from build123d import *

# Parameters (mm, degrees)
SKETCH1_R                      = 29.464
BASE_DEPTH                     = 25.4
SKETCH2_W                      = 33.02
SKETCH2_H                      = 3.81
A_ARMS_DEPTH                   = 25.4
FILLET_A_ARM_TAB_F_R           = 16.51
FILLET2_R                      = 50.8
BOSS_EXTRUDE3_DEPTH            = 10
FILLET3_R                      = 12.7
SKETCH6_R                      = 4.064
TAB_HOLES_1_DEPTH              = 38.1
SKETCH7_R                      = 4.064
TAB_HOLES_2_DEPTH              = 177.509801452
MID_FEATURE_BEARING_DEPTH      = 1.524
MID_FEATURE_BEARING_DEPTH_BACK = 1.524
SKETCH8_R                      = 29.464
SKETCH8_R_2                    = 26.924
SKETCH11_R                     = 4.318
TAB_HOLES_3_DEPTH              = 50.8


with BuildPart() as part:
    # Sketch1 → Base (new body)
    with BuildSketch(Plane(origin=(0, 0, 0), x_dir=(1, 0, 0), z_dir=(0, 1, 0))):
        with BuildLine():
            Line((-58.88559997, -79.728413598), (36.107103946, -79.728413598))
            Line((36.107103946, -79.728413598), (42.479503863, -4.99030836))
            Line((42.479503863, -4.99030836), (36.107103946, 103.339537331))
            Line((36.107103946, 103.339537331), (9.149946216, 103.339537331))
            ThreePointArc((9.149946216, 103.339537331), (-6.239768533, 98.146384684), (-15.336480298, 84.690457011))
            Line((-15.336480298, 84.690457011), (-53.313910816, -53.058413598))
            Line((-53.313910816, -53.058413598), (-58.88559997, -53.058413598))
            Line((-58.88559997, -53.058413598), (-58.88559997, -79.728413598))
        make_face()
        with Locations(Location((0, 0, 0), (0, 0, 270))):
            Circle(SKETCH1_R, mode=Mode.SUBTRACT)
    extrude(amount=BASE_DEPTH)

    # Sketch2 → A-Arms (add)
    with BuildSketch(Plane(origin=(0, 0, 0), x_dir=(1, 0, 0), z_dir=(0, 1, 0))):
        Polygon((36.107103946, 103.339537331), (36.331223565, 99.529537331), (3.087103946, 99.529537331), (3.087103946, 103.339537331), align=None)
        Polygon((3.087103946, -75.918413598), (36.431956223, -75.918413598), (36.107103946, -79.728413598), (3.087103946, -79.728413598), align=None)
        Polygon((3.087103946, 80.479537331), (3.087103946, 76.669537331), (37.675941275, 76.669537331), (37.451821657, 80.479537331), align=None)
        Polygon((3.087103946, -53.058413598), (38.381069887, -53.058413598), (38.056217609, -56.868413598), (3.087103946, -56.868413598), align=None)
        with Locations((-42.37559997, -54.963413598)):
            Rectangle(SKETCH2_W, SKETCH2_H)
        with Locations((-42.37559997, -77.823413598)):
            Rectangle(SKETCH2_W, SKETCH2_H)
    extrude(amount=-A_ARMS_DEPTH)

    # Fillet a-arm tab f
    # the kernel refuses this fillet: 16.51 mm, written as the material it takes off along each edge
    with BuildSketch(Plane(origin=(39.93846651, -25.4, 34.792630802), x_dir=(-0.9963848042708363, 0, -0.08495482221844149), z_dir=(-0.08495482221844149, 0, 0.9963848042708364)), Plane(origin=(41.887580174, -25.4, 11.932630802), x_dir=(-0.9963848042708365, 0, -0.08495482221843932), z_dir=(-0.08495482221843934, 0, 0.9963848042708366))) as fillet_a_arm_tab_f_piece_1:
        with BuildLine():
            CenterArc((FILLET_A_ARM_TAB_F_R, -FILLET_A_ARM_TAB_F_R), FILLET_A_ARM_TAB_F_R, 90, 90)
            Line((0, -FILLET_A_ARM_TAB_F_R), (0, 0))
            Line((0, 0), (FILLET_A_ARM_TAB_F_R, 0))
        make_face()
    extrude(amount=86.373823872, mode=Mode.SUBTRACT)
    with BuildSketch(Plane(origin=(3.087103946, -25.4, 121.003413598), x_dir=(0, 1, 0), z_dir=(0, 0, -1)), Plane(origin=(3.087103946, -25.4, -121.754537331), x_dir=(1, 0, 0), z_dir=(0, 0, 1)), Plane(origin=(-25.86559997, -25.4, 98.143413598), x_dir=(-1, 0, 0), z_dir=(0, 0, -1)), Plane(origin=(-58.88559997, -25.4, 11.783413598), x_dir=(1, 0, 0), z_dir=(0, 0, 1))) as fillet_a_arm_tab_f_piece_2:
        with BuildLine():
            CenterArc((FILLET_A_ARM_TAB_F_R, FILLET_A_ARM_TAB_F_R), FILLET_A_ARM_TAB_F_R, 180, 90)
            Line((0, FILLET_A_ARM_TAB_F_R), (0, 0))
            Line((0, 0), (FILLET_A_ARM_TAB_F_R, 0))
        make_face()
    extrude(amount=86.36, mode=Mode.SUBTRACT)
    with BuildSketch(Plane(origin=(3.087103946, -25.4, 98.143413598), x_dir=(1, 0, 0), z_dir=(0, 0, -1)), Plane(origin=(3.087103946, -25.4, -58.254537331), x_dir=(1, 0, 0), z_dir=(0, 0, -1)), Plane(origin=(-58.88559997, -25.4, 121.003413598), x_dir=(1, 0, 0), z_dir=(0, 0, -1)), Plane(origin=(-25.86559997, -25.4, 34.643413598), x_dir=(-1, 0, 0), z_dir=(0, 0, 1))) as fillet_a_arm_tab_f_piece_3:
        with BuildLine():
            CenterArc((FILLET_A_ARM_TAB_F_R, -FILLET_A_ARM_TAB_F_R), FILLET_A_ARM_TAB_F_R, 90, 90)
            Line((0, -FILLET_A_ARM_TAB_F_R), (0, 0))
            Line((0, 0), (FILLET_A_ARM_TAB_F_R, 0))
        make_face()
    extrude(amount=86.36, mode=Mode.SUBTRACT)
    with BuildSketch(Plane(origin=(40.099713977, -25.4, -35.465763828), x_dir=(-0.9982743428955775, 0, 0.05872253669931843), z_dir=(-0.05872253669931843, 0, -0.9982743428955776)), Plane(origin=(33.683331244, -25.4, -144.543310834), x_dir=(0, 1, 0), z_dir=(0.05872253669931843, 0, 0.9982743428955776))) as fillet_a_arm_tab_f_piece_4:
        with BuildLine():
            CenterArc((FILLET_A_ARM_TAB_F_R, FILLET_A_ARM_TAB_F_R), FILLET_A_ARM_TAB_F_R, 180, 90)
            Line((0, FILLET_A_ARM_TAB_F_R), (0, 0))
            Line((0, 0), (FILLET_A_ARM_TAB_F_R, 0))
        make_face()
    extrude(amount=86.366586119, mode=Mode.SUBTRACT)

    # Fillet2
    fillet2_edges = [part.edges().sort_by_distance(p)[0] for p in [
        (42.479503863, 12.7, 4.99030836),
    ]]
    fillet(fillet2_edges, radius=FILLET2_R)

    # Sketch3 → Boss-Extrude3 (add)
    with BuildSketch(Plane(origin=(0, 25.4, 0), x_dir=(-1, 0, 0), z_dir=(0, -1, 0))):
        with BuildLine():
            Line((47.666796836, 52.78191811), (25.796089041, 46.75215335))
            Line((25.796089041, 46.75215335), (45.913565896, -26.216440853))
            Line((45.913565896, -26.216440853), (68.231322711, -20.063424462))
            ThreePointArc((68.231322711, -20.063424462), (68.827916005, -17.910119441), (69.356571433, -15.739135906))
            ThreePointArc((69.356571433, -15.739135906), (66.028611601, -10.941366051), (70.726242467, -7.473488245))
            ThreePointArc((70.726242467, -7.473488245), (70.885962372, -5.764957818), (71.004415449, -4.053071275))
            ThreePointArc((71.004415449, -4.053071275), (70.020531637, -4.0078353), (69.039031874, -4.089883254))
            ThreePointArc((69.039031874, -4.089883254), (65.518990894, -3.323443269), (63.392280792, -0.415656673))
            Line((63.392280792, -0.415656673), (54.014483076, 33.598783658))
            ThreePointArc((54.014483076, 33.598783658), (54.320283062, 37.122596493), (56.852004495, 39.592648541))
            ThreePointArc((56.852004495, 39.592648541), (57.672230058, 40.01773376), (58.434985849, 40.538954462))
            ThreePointArc((58.434985849, 40.538954462), (57.439925969, 41.936968234), (56.41142698, 43.310568065))
            ThreePointArc((56.41142698, 43.310568065), (50.594219677, 43.814563519), (50.926596454, 49.644095052))
            ThreePointArc((50.926596454, 49.644095052), (49.321656334, 51.238936528), (47.666796836, 52.78191811))
        make_face()
        with BuildLine():
            Line((51.737082765, 53.904097917), (47.666796836, 52.78191811))
            ThreePointArc((47.666796836, 52.78191811), (49.321656334, 51.238936528), (50.926596454, 49.644095052))
            ThreePointArc((50.926596454, 49.644095052), (55.447559185, 50.395432037), (57.95335867, 46.558169963))
            ThreePointArc((57.95335867, 46.558169963), (57.548301504, 44.760638918), (56.41142698, 43.310568065))
            ThreePointArc((56.41142698, 43.310568065), (57.439925969, 41.936968234), (58.434985849, 40.538954462))
            ThreePointArc((58.434985849, 40.538954462), (60.574765152, 49.972187818), (51.737082765, 53.904097917))
        make_face()
        with BuildLine():
            ThreePointArc((69.356571433, -15.739135906), (68.827916005, -17.910119441), (68.231322711, -20.063424462))
            Line((68.231322711, -20.063424462), (72.188506448, -18.972426984))
            ThreePointArc((72.188506448, -18.972426984), (77.759344227, -11.023625151), (71.004415449, -4.053071275))
            ThreePointArc((71.004415449, -4.053071275), (70.885962372, -5.764957818), (70.726242467, -7.473488245))
            ThreePointArc((70.726242467, -7.473488245), (73.319499224, -8.869245139), (74.354230544, -11.62649903))
            ThreePointArc((74.354230544, -11.62649903), (72.826290125, -14.862637881), (69.356571433, -15.739135906))
        make_face()
    extrude(amount=BOSS_EXTRUDE3_DEPTH)

    # Fillet3
    fillet3_edges = [part.edges().sort_by_distance(p)[0] for p in [
        (-25.796089041, 20.4, -46.75215335),
        (-45.913565896, 20.4, 26.216440853),
    ]]
    fillet(fillet3_edges, radius=FILLET3_R)

    # Sketch6 → Tab Holes 1 (cut)
    with BuildSketch(Plane(origin=(0, 0, -103.339537331), x_dir=(-1, 0, 0), z_dir=(0, 0, -1))):
        with Locations((-19.582846345, -11.893705932)):
            Circle(SKETCH6_R)
    extrude(amount=-TAB_HOLES_1_DEPTH, mode=Mode.SUBTRACT)

    # Sketch7 → Tab Holes 2 (cut, through all)
    with BuildSketch(Plane(origin=(0, 0, 53.058413598), x_dir=(-1, 0, 0), z_dir=(0, 0, -1))):
        with Locations((42.37559997, -16.51)):
            Circle(SKETCH7_R)
    extrude(amount=-TAB_HOLES_2_DEPTH, mode=Mode.SUBTRACT)

    # Sketch8 → mid-feature bearing (add, two sides: drawn at the far end of the back side and taken through both)
    with BuildSketch(Plane(origin=(0, 12.7, 0), x_dir=(1, 0, 0), z_dir=(0, 1, 0)).offset(-MID_FEATURE_BEARING_DEPTH_BACK)):
        with Locations(Location((0, 0, 0), (0, 0, 270))):
            Circle(SKETCH8_R)
        with Locations(Location((0, 0, 0), (0, 0, 270))):
            Circle(SKETCH8_R_2, mode=Mode.SUBTRACT)
    extrude(amount=MID_FEATURE_BEARING_DEPTH + MID_FEATURE_BEARING_DEPTH_BACK)

    # Sketch11 → Tab Holes 3 (cut)
    with BuildSketch(Plane(origin=(0, 0, 79.728413598), x_dir=(-1, 0, 0), z_dir=(0, 0, -1))):
        with Locations(Location((-19.862052779, -16.51, 0), (0, 0, 180))):
            Circle(SKETCH11_R)
    extrude(amount=TAB_HOLES_3_DEPTH, mode=Mode.SUBTRACT)


solid = part.part
Build history of the part. All positions in model axes, mm. A direction names the side the tool comes from. Round coordinates to 2 decimals unless told otherwise and drop trailing zeros. Loops run counter-clockwise (first coordinate to the right, second up) from the corner with the lowest first, then second, coordinate; pieces in that order, holes last. Notation, with made-up numbers: (-23, 2.5) -> (35, 2.5) arc R23 ccw to (35, 41.5) -> close; hole circle Ø7 at (29, -27). An arc over 180 degrees is marked (long way). Answer in a Markdown table with one row per item.
Item 1: Drill centre lines: L1, parallel to Z at x = 31, y = -10; L2, parallel to Z at x = -46.5, y = -5; L3, parallel to Z at x = -2, y = 22. Where is each one in solid material? Low to high. Write a range as [from, to].
Answers below:
| item | result |
|---|---|
| L1 | z = [-103.34, -99.53], [-80.48, -76.67], [53.06, 56.87], [75.92, 79.73] |
| L2 | z = [53.06, 56.87], [75.92, 79.73] |
| L3 | z = [-100.76, -29.4], [29.4, 79.73] |
Item 2: Saw through at A-A (y = -2). Write the cut outline in (x, z), and give its area (3 significant figures).
Answers below:
| item | result |
|---|---|
| outline | (-58.89, 53.06) -> (-25.87, 53.06) -> (-25.87, 56.87) -> (-58.89, 56.87) -> close; (-58.89, 75.92) -> (-25.87, 75.92) -> (-25.87, 79.73) -> (-58.89, 79.73) -> close; (3.09, -103.34) -> (36.11, -103.34) -> (36.33, -99.53) -> (3.09, -99.53) -> close; (3.09, -80.48) -> (37.45, -80.48) -> (37.68, -76.67) -> (3.09, -76.67) -> close; (3.09, 53.06) -> (38.38, 53.06) -> (38.06, 56.87) -> (3.09, 56.87) -> close; (3.09, 75.92) -> (36.43, 75.92) -> (36.11, 79.73) -> (3.09, 79.73) -> close |
| area | 769 mm² |
Item 3: Saw through at B-B (y = 19.5). Write the cut outline in (x, z), and give its area (3 significant figures).
Answers below:
| item | result |
|---|---|
| outline | (-72.19, 18.97) arc R7.62 ccw to (-69.04, 4.09) arc R5.08 cw to (-63.39, 0.42) -> (-54.01, -33.6) arc R5.08 cw to (-56.85, -39.59) arc R7.62 ccw to (-51.74, -53.9) -> (-38.04, -50.13) arc R12.7 cw to (-22.42, -59) -> (-15.34, -84.69) arc R25.4 ccw to (9.15, -103.34) -> (36.11, -103.34) -> (42.26, 1.34) arc R50.8 ccw to (42.17, 8.64) -> (36.11, 79.73) -> (-58.89, 79.73) -> (-58.89, 53.06) -> (-53.31, 53.06) -> (-49.29, 38.46) arc R12.7 cw to (-58.16, 22.84) -> close; hole circle Ø8.38 at (-70.16, 11.63); hole circle Ø8.38 at (-53.76, -46.56); hole circle Ø58.93 at (0, 0) |
| area | 13,000 mm² |
Item 4: Saw through at C-C (z = -73). Write the cut outline in (x, y), and give its area (3 significant figures).
Answers below:
| item | result |
|---|---|
| outline | (-18.56, 0) -> (37.89, 0) -> (37.89, 25.4) -> (-18.56, 25.4) -> close |
| area | 1,430 mm² |
Item 5: Pin check, flat tips, straight feed: pin 1 (14 mm diameter, centred on x = 19.86, y = -16.51, fed in from +Z); pin 2 (8 mm diameter, centred on y = 6, z = 69, fed in from -X); pin 3 (3 mm diameter, centred on y = -3, z = -79, fed in from -X); pin 4 (3 mm diameter, centred on y = -5, z = 54, fed in from +X). Stop position of each tip, or through.
Answers below:
| item | result |
|---|---|
| pin 1 | stops at z = 79.73 |
| pin 2 | stops at x = -58.89 |
| pin 3 | stops at x = 3.09 |
| pin 4 | stops at x = 38.38 |
Item 6: Which spindle directions (+Z, -Z, +X, -X, +Y, -Y) get a long thin tool onto all of the face, cutting with end or side? Do faces 4 (the flat face through (-25.866, -4, 78)), 5 (the flat face through (-24, 11.176, 13)), 6 (the flat face through (21, -10, 56.868)). Say none if no direction does.
Answers below:
| item | result |
|---|---|
| face 4 | +Z, -Z, -Y |
| face 5 | -Y |
| face 6 | +X, -X, -Y |
Item 7: Mould opens along Z. For faces 1 (the cylindrical face through (-65.56, 20.47, 3.35)), 2 (the flat face through (24, -13, -99.53)), 3 (the cylindrical face through (8.05, -20.69, 54.99)) say: +Z half, -Z half, draft (parallel to the pull), parting line (faces both ways), or undercut.
Answers below:
| item | result |
|---|---|
| face 1 | -Z half |
| face 2 | undercut |
| face 3 | draft |
